The listing builds one solid part. Answer for the finished solid, in the listing's coordinates (mm). Give positions to 0.01 mm unless a question says otherwise; leave off trailing zeros. Loops run counter-clockwise (first coordinate to the right, second up) from the corner with the lowest first, then second, coordinate; pieces in that order, holes last. Notation, with made-up numbers: M -29.5,86 L 8.5,86 A13 cw 8.5,98 Z; hole C 84,-15 d6. An arc over 180 degrees is marked long. One line per item, written item: value. Start each with the question number.
Q1. Flat-ended cylindrical pins translate along their axes: pin 1 (8 mm diameter, centred on x = -4.5, y = 9.5, fed in from +Z); pin 2 (2 mm diameter, centred on y = -3.5, z = 2.5, fed in from -X). Find the tip coordinate at first contact, or state that the pin passes through.
Q2. A cutting plane is placed at D-D, the plane z = 3.9. Determine the outline of the cut face in (x, y).
Q3. Consider L1, parallel to Y at x = 0, z = 1.65; L2, parallel to Z at x = 6, y = 11.5; L3, parallel to Y at x = 1.25, z = 1.95. Determine where each line is inside the solid, lowest interval first.
Q4. A cutting plane is placed at C-C, the plane z = 0.5. Determine the outline of the cut face in (x, y), and give its area (3 significant figures).
Q5. The mould has two halves that part along X. Classify faces 1 (the cylindrical face through (-0.325, 5.536, 1.014)), 2 (the flat face through (0, 4, 2)), 3 (the cylindrical face through (-8.5, 0.07, 1.01)), 4 (the cylindrical face through (-3, 0, 3)): +X half, -X half, draft (parallel to the pull), parting line (faces both ways), or undercut.
Q6. A cutting plane is placed at A-A, the plane x = -7. Determine the outline of the cut face in (y, z).
from build123d import *

# Parameters (mm, degrees)
SKETCH_1_R               = 15
EXTRUDE_1_DEPTH          = 2
SKETCH_2_R               = 3
SKETCH_2_R_2             = 1
EXTRUDE_2_DEPTH          = 2.3
SKETCH_3_R               = 1
CUT_EXTRUDE_1_DEPTH      = 6
SKETCH_4_R               = 1
CUT_EXTRUDE_2_DEPTH      = 22.644629819
SKETCH_5_R               = 1.5
CUT_EXTRUDE_3_DEPTH      = 10
CUT_EXTRUDE_4_DEPTH      = 2
CUT_EXTRUDE_4_DEPTH_BACK = 1.1
SKETCH_6_R               = 0.4


with BuildPart() as part:
    # 草图1 → 凸台-拉伸1 (new body)
    with BuildSketch(Plane.XY):
        Circle(SKETCH_1_R)
    extrude(amount=EXTRUDE_1_DEPTH)

    # 草图2 → 凸台-拉伸2 (add)
    with BuildSketch(Plane.XY.offset(2)):
        Circle(SKETCH_2_R)
        Circle(SKETCH_2_R_2, mode=Mode.SUBTRACT)
    extrude(amount=EXTRUDE_2_DEPTH)

    # 草图3 → 切除-拉伸1 (cut)
    with BuildSketch(Plane.XY.offset(2)):
        with Locations((0, 7)):
            Circle(SKETCH_3_R)
        with Locations((7, 0)):
            Circle(SKETCH_3_R)
        with Locations((0, -7)):
            Circle(SKETCH_3_R)
        with Locations((-7, 0)):
            Circle(SKETCH_3_R)
    extrude(amount=-CUT_EXTRUDE_1_DEPTH, mode=Mode.SUBTRACT)

    # 草图4 → 切除-拉伸2 (cut, through all)
    with BuildSketch(Plane(origin=(0, 0, 0), x_dir=(-1, 0, 0), z_dir=(0, 0, -1))):
        Circle(SKETCH_4_R)
    extrude(amount=-CUT_EXTRUDE_2_DEPTH, mode=Mode.SUBTRACT)

    # 草图5 → 切除-拉伸3 (cut)
    with BuildSketch(Plane.XY.offset(2)):
        with Locations((0, 7)):
            Circle(SKETCH_5_R)
        with Locations((-7, 0)):
            Circle(SKETCH_5_R)
        with Locations((7, 0)):
            Circle(SKETCH_5_R)
        with Locations((0, -7)):
            Circle(SKETCH_5_R)
    extrude(amount=-CUT_EXTRUDE_3_DEPTH, mode=Mode.SUBTRACT)

    # 草图6 → 切除-拉伸4 (cut, two sides: drawn at the far end of the back side and taken through both)
    with BuildSketch(Plane(origin=(64.521548832, -12.754908116, 46.976284772), x_dir=(0, 0, -1), z_dir=(-0.22357508845081375, -0.9746867085500914, 1.0628725110972871e-14)).offset(-CUT_EXTRUDE_4_DEPTH_BACK)):
        with Locations(Location((43.872176256, -65.74, 0), (0, 0, 270))):
            Circle(SKETCH_6_R)
    extrude(amount=CUT_EXTRUDE_4_DEPTH + CUT_EXTRUDE_4_DEPTH_BACK, mode=Mode.SUBTRACT)


solid = part.part
Answer block:
1. pin 1: z = 2
1. pin 2: x = -14.77
2. outline: C 0,0 d6; hole C 0,0 d2
3. L1: -15 to -8.5, -5.5 to -1, 1 to 5.5, 8.5 to 15
3. L2: 0 to 2
3. L3: -14.95 to -7.83, -6.17 to 6.17, 7.83 to 14.95
4. outline: C 0,0 d30; hole C -7,0 d3; hole C 0,-7 d3; hole C 0,7 d3; hole C 0,0 d2; hole C 7,0 d3
4. area: 675 mm^2
5. face 1: undercut
5. face 2: draft
5. face 3: undercut
5. face 4: parting line
6. outline: M -13.27,0 L -1.5,0 L -1.5,2 L -13.27,2 Z; M 1.5,0 L 13.27,0 L 13.27,2 L 1.5,2 Z
